For this review, take the finished solid that the model builds, in its own axes (mm). Face numbers are marked on the shaded views. A direction names the side the tool comes from. Coordinates: 2 decimals unless noted, no trailing zeros. Write each loop counter-clockwise with the first axis right and the second up, starting at its lowest first coordinate (ties: lowest second). Pieces come first, ordered by that corner, then holes. Notation, with made-up numbers: M 24,71.25 L 46,71.25 A17 ccw 46,97.25 Z; hole C 80,-23.5 d3. An arc over 180 degrees is marked long. One line per question, with ' | ' between items.
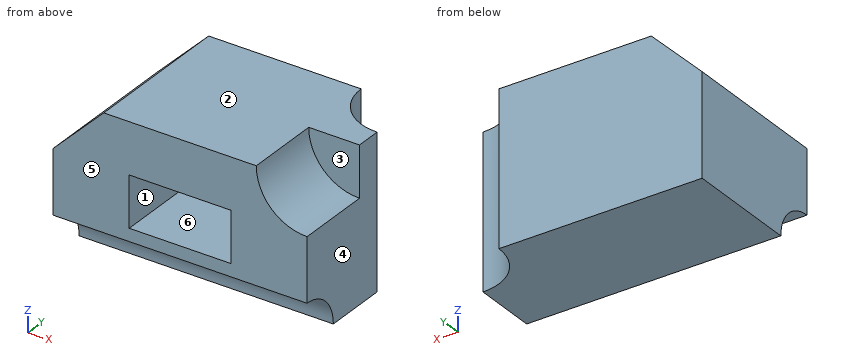
from build123d import *

# Parameters (mm, degrees)
F0_W      = 50
F0_H      = 30
F1_DEPTH  = 30
F3_DEPTH  = 30.001
F4_R      = 10
F5_DEPTH  = 15
F6_W      = 20
F6_H      = 10
F7_DEPTH  = 20
F8_R      = 7.5
F9_DEPTH  = 50.001
F10_R     = 10
F11_DEPTH = 30.001


with BuildPart() as f1:
    # F0 (on Top) → F1 (new body)
    with BuildSketch(Plane.XY):
        with Locations((25, 15)):
            Rectangle(F0_W, F0_H)
    extrude(amount=F1_DEPTH)

    # F2 (on face) → F3 (cut, through all)
    with BuildSketch(Plane.XZ):
        Polygon((10, 30), (0, 30), (0, 20), align=None)
    extrude(amount=-F3_DEPTH, mode=Mode.SUBTRACT)

    # F4 (on face) → F5 (cut)
    with BuildSketch(Plane.XZ):
        with Locations((50, 30)):
            Circle(F4_R)
    extrude(amount=-F5_DEPTH, mode=Mode.SUBTRACT)

    # F6 (on face) → F7 (cut)
    with BuildSketch(Plane.XZ):
        with Locations((25, 15)):
            Rectangle(F6_W, F6_H)
    extrude(amount=-F7_DEPTH, mode=Mode.SUBTRACT)

    # F8 (on face) → F9 (cut, through all)
    with BuildSketch(Plane.YZ.offset(50)):
        Circle(F8_R)
    extrude(amount=-F9_DEPTH, mode=Mode.SUBTRACT)

    # F10 (on face) → F11 (cut, through all)
    with BuildSketch(Plane.XY.offset(30)):
        with Locations((50, 30)):
            Circle(F10_R)
    extrude(amount=-F11_DEPTH, mode=Mode.SUBTRACT)


solid = f1.part
1) We need section D-D on y = 19. State the section outline as (x, z) points.
Responses:
outline: M 0,0 L 50,0 L 50,30 L 10,30 L 0,20 Z; hole M 15,10 L 35,10 L 35,20 L 15,20 Z
2) To check wall thickness, follow line 1 along Z through (x, y) = (34, 11.5); line 2 along Y through (x, z) = (34.5, 12.5); line 3 along X through (y, z) = (12.5, 16). State the ranges of each line that lie inside material, in increasing order. Write a range as [from, to].
Responses:
line 1: [0, 10], [20, 30] | line 2: [20, 30] | line 3: [0, 15], [35, 50]
3) Insertion check: pin 1 Ø5 at (x, z) = (23.5, 15) entering from -Y; pin 2 Ø3 at (x, z) = (45.5, 23.5) entering from -Y. Each pin has a flat end and moves straight along its axis. Give the tip position at first contact, or say it passes through.
Responses:
pin 1: y = 20 | pin 2: y = 15
4) Machinability: for the marked faces 1, 2 and 3, which of the approach directions +Z, -Z, +X, -X, +Y, -Y give a long, thin tool a straight path to every point of the face, cutting with its end or side? Answer none if there is none.
Responses:
face 1: -Y | face 2: +Z, +X, -X, +Y, -Y | face 3: +Z, +X, -Y
5) The part is to be moulded in two halves that separate along X. For the marked faces 4, 5 and 6, say which applies: +X half, -X half, draft (parallel to the pull), parting line (faces both ways), or undercut.
Responses:
face 4: +X half | face 5: draft | face 6: undercut
6) We need section A-A on y = 13. State the section outline as (x, z) points.
Responses:
outline: M 0,0 L 50,0 L 50,20 A10 cw 40,30 L 10,30 L 0,20 Z; hole M 15,10 L 35,10 L 35,20 L 15,20 Z
7) We need section C-C on z = 15.5. State the section outline as (x, y) points.
Responses:
outline: M 0,0 L 15,0 L 15,20 L 35,20 L 35,0 L 50,0 L 50,20 A10 cw 40,30 L 0,30 Z
8) We need section B-B on x = 19. State the section outline as (y, z) points.
Responses:
outline: M 0,7.5 A7.5 cw 7.5,0 L 30,0 L 30,30 L 0,30 L 0,20 L 20,20 L 20,10 L 0,10 Z
